from build123d import *

# Parameters (mm, degrees)
SKETCH1_W               = 298.45
SKETCH1_H               = 76.2
BOSS_EXTRUDE1_DEPTH     = 6.35
SKETCH2_W               = 12.7
SKETCH2_H               = 25.4
CUT_EXTRUDE5_DEPTH      = 155.142898393
LPATTERN1_COUNT         = 9
LPATTERN1_PITCH         = 25.4
MIRROR1_COPY_1_SKETCH_W = 12.7
MIRROR1_COPY_1_SKETCH_H = 25.4
MIRROR1_COPY_1_DEPTH    = 155.142898393
MIRROR1_COPY_2_SKETCH_W = 12.7
MIRROR1_COPY_2_SKETCH_H = 25.4
MIRROR1_COPY_2_DEPTH    = 155.142898393
MIRROR1_COPY_3_SKETCH_W = 12.7
MIRROR1_COPY_3_SKETCH_H = 25.4
MIRROR1_COPY_3_DEPTH    = 155.142898393
MIRROR1_COPY_4_SKETCH_W = 12.7
MIRROR1_COPY_4_SKETCH_H = 25.4
MIRROR1_COPY_4_DEPTH    = 155.142898393
MIRROR1_COPY_5_SKETCH_W = 12.7
MIRROR1_COPY_5_SKETCH_H = 25.4
MIRROR1_COPY_5_DEPTH    = 155.142898393
MIRROR1_COPY_6_SKETCH_W = 12.7
MIRROR1_COPY_6_SKETCH_H = 25.4
MIRROR1_COPY_6_DEPTH    = 155.142898393
MIRROR1_COPY_7_SKETCH_W = 12.7
MIRROR1_COPY_7_SKETCH_H = 25.4
MIRROR1_COPY_7_DEPTH    = 155.142898393
MIRROR1_COPY_8_SKETCH_W = 12.7
MIRROR1_COPY_8_SKETCH_H = 25.4
MIRROR1_COPY_8_DEPTH    = 155.142898393
SKETCH3_W               = 40.748476415
SKETCH3_H               = 6.35
SKETCH3_W_2             = 25.4
SKETCH3_H_2             = 9.525
CUT_EXTRUDE7_DEPTH      = 155.142898393
SKETCH4_W               = 15.875
SKETCH4_H               = 25.4
CUT_EXTRUDE8_DEPTH      = 155.142898393


with BuildPart() as part:
    # Sketch1 → Boss-Extrude1 (new body)
    with BuildSketch(Plane.XY):
        Rectangle(SKETCH1_W, SKETCH1_H)
    extrude(amount=BOSS_EXTRUDE1_DEPTH)

    # Sketch2 → Cut-Extrude5 (cut, symmetric)
    with BuildSketch(Plane.XY):
        with Locations((101.6, -44.45)):
            Rectangle(SKETCH2_W, SKETCH2_H)
    cut_extrude5 = extrude(amount=CUT_EXTRUDE5_DEPTH, both=True, mode=Mode.SUBTRACT)

    # LPattern1: Cut-Extrude5 ×9
    with Locations(*[(-i * LPATTERN1_PITCH, 0, 0) for i in range(1, LPATTERN1_COUNT)]):
        add(cut_extrude5, mode=Mode.SUBTRACT)

    # Mirror1: Cut-Extrude5 across plane
    add(cut_extrude5.mirror(Plane.ZX), mode=Mode.SUBTRACT)

    # Mirror1 copy 1 sketch → Mirror1 copy 1 (cut, symmetric)
    with BuildSketch(Plane(origin=(-25.4, 0, 0), x_dir=(1, 0, 0), z_dir=(0, 0, 1))):
        with Locations((101.6, 44.45)):
            Rectangle(MIRROR1_COPY_1_SKETCH_W, MIRROR1_COPY_1_SKETCH_H)
    extrude(amount=MIRROR1_COPY_1_DEPTH, both=True, mode=Mode.SUBTRACT)

    # Mirror1 copy 2 sketch → Mirror1 copy 2 (cut, symmetric)
    with BuildSketch(Plane(origin=(-50.8, 0, 0), x_dir=(1, 0, 0), z_dir=(0, 0, 1))):
        with Locations((101.6, 44.45)):
            Rectangle(MIRROR1_COPY_2_SKETCH_W, MIRROR1_COPY_2_SKETCH_H)
    extrude(amount=MIRROR1_COPY_2_DEPTH, both=True, mode=Mode.SUBTRACT)

    # Mirror1 copy 3 sketch → Mirror1 copy 3 (cut, symmetric)
    with BuildSketch(Plane(origin=(-76.2, 0, 0), x_dir=(1, 0, 0), z_dir=(0, 0, 1))):
        with Locations((101.6, 44.45)):
            Rectangle(MIRROR1_COPY_3_SKETCH_W, MIRROR1_COPY_3_SKETCH_H)
    extrude(amount=MIRROR1_COPY_3_DEPTH, both=True, mode=Mode.SUBTRACT)

    # Mirror1 copy 4 sketch → Mirror1 copy 4 (cut, symmetric)
    with BuildSketch(Plane(origin=(-101.6, 0, 0), x_dir=(1, 0, 0), z_dir=(0, 0, 1))):
        with Locations((101.6, 44.45)):
            Rectangle(MIRROR1_COPY_4_SKETCH_W, MIRROR1_COPY_4_SKETCH_H)
    extrude(amount=MIRROR1_COPY_4_DEPTH, both=True, mode=Mode.SUBTRACT)

    # Mirror1 copy 5 sketch → Mirror1 copy 5 (cut, symmetric)
    with BuildSketch(Plane(origin=(-127, 0, 0), x_dir=(1, 0, 0), z_dir=(0, 0, 1))):
        with Locations((101.6, 44.45)):
            Rectangle(MIRROR1_COPY_5_SKETCH_W, MIRROR1_COPY_5_SKETCH_H)
    extrude(amount=MIRROR1_COPY_5_DEPTH, both=True, mode=Mode.SUBTRACT)

    # Mirror1 copy 6 sketch → Mirror1 copy 6 (cut, symmetric)
    with BuildSketch(Plane(origin=(-152.4, 0, 0), x_dir=(1, 0, 0), z_dir=(0, 0, 1))):
        with Locations((101.6, 44.45)):
            Rectangle(MIRROR1_COPY_6_SKETCH_W, MIRROR1_COPY_6_SKETCH_H)
    extrude(amount=MIRROR1_COPY_6_DEPTH, both=True, mode=Mode.SUBTRACT)

    # Mirror1 copy 7 sketch → Mirror1 copy 7 (cut, symmetric)
    with BuildSketch(Plane(origin=(-177.8, 0, 0), x_dir=(1, 0, 0), z_dir=(0, 0, 1))):
        with Locations((101.6, 44.45)):
            Rectangle(MIRROR1_COPY_7_SKETCH_W, MIRROR1_COPY_7_SKETCH_H)
    extrude(amount=MIRROR1_COPY_7_DEPTH, both=True, mode=Mode.SUBTRACT)

    # Mirror1 copy 8 sketch → Mirror1 copy 8 (cut, symmetric)
    with BuildSketch(Plane(origin=(-203.2, 0, 0), x_dir=(1, 0, 0), z_dir=(0, 0, 1))):
        with Locations((101.6, 44.45)):
            Rectangle(MIRROR1_COPY_8_SKETCH_W, MIRROR1_COPY_8_SKETCH_H)
    extrude(amount=MIRROR1_COPY_8_DEPTH, both=True, mode=Mode.SUBTRACT)

    # Sketch3 → Cut-Extrude7 (cut, through all)
    with BuildSketch(Plane.XY):
        with Locations((163.249238208, 12.7)):
            Rectangle(SKETCH3_W, SKETCH3_H)
        with Locations((163.249238208, 0)):
            Rectangle(SKETCH3_W, SKETCH3_H)
        with Locations((163.249238208, -12.7)):
            Rectangle(SKETCH3_W, SKETCH3_H)
        with Locations((155.575, 26.9875)):
            Rectangle(SKETCH3_W_2, SKETCH3_H_2)
        with Locations((155.575, -26.9875)):
            Rectangle(SKETCH3_W_2, SKETCH3_H_2)
    cut_extrude7 = extrude(amount=CUT_EXTRUDE7_DEPTH, mode=Mode.SUBTRACT)

    # Mirror2: Cut-Extrude7 across plane
    add(cut_extrude7.mirror(Plane(origin=(0, 0, 0), x_dir=(0, 0, 1), z_dir=(1, 0, 0))), mode=Mode.SUBTRACT)

    # Sketch4 → Cut-Extrude8 (cut, through all)
    with BuildSketch(Plane.XY.offset(6.35)):
        with Locations((128.5875, -44.45)):
            Rectangle(SKETCH4_W, SKETCH4_H)
        with Locations((-128.5875, -44.45)):
            Rectangle(SKETCH4_W, SKETCH4_H)
        with Locations((-128.5875, 44.45)):
            Rectangle(SKETCH4_W, SKETCH4_H)
        with Locations((128.5875, 44.45)):
            Rectangle(SKETCH4_W, SKETCH4_H)
    extrude(amount=-CUT_EXTRUDE8_DEPTH, mode=Mode.SUBTRACT)


solid = part.part
Work out the finished part from the listing and answer in its coordinate system (mm). A direction names the side the tool comes from. Give positions to 0.01 mm unless a question says otherwise; leave off trailing zeros. Loops run counter-clockwise (first coordinate to the right, second up) from the corner with the lowest first, then second, coordinate; pieces in that order, holes last. Notation, with made-up numbers: (-3, -25.5) -> (19, -25.5) arc R17 cw to (19, 2.5) -> close; hole circle Ø1 at (-25.75, 4). An arc over 180 degrees is marked (long way). Use a Markdown table: item, result. Add a question column.
1. Section A-A on y = -12.5 is taken. Determine the outline of the cut face in (x, z) (3 decimals).
2. Section B-B on x = 28.5 is taken. Determine the outline of the cut face in (y, z), and give its area (3 significant figures).
3. For faces 1 (the flat face through (146, -3.175, 3)), 2 (the flat face through (95.25, 35, 3)), 3 (the flat face through (-25, -31.75, 3)), 4 (the flat face through (-146, 22.225, 3)), determine the directions among +Z, -Z, +X, -X, +Y, -Y from which every point of the face is accessible in a straight line to the end or side of a thin tool.
4. Find the intervals of material crossed by probe 1 along Y at (x, z) = (-3.5, 3.75); probe 2 along X at (y, z) = (30.5, 5) (3 decimals), in increasing order.
5. Flat-ended cylindrical pins translate along their axes: pin 1 Ø3 at (x, y) = (24.5, -14) entering from -Z; pin 2 Ø3 at (x, z) = (-126.5, 4) entering from +Y; pin 3 Ø3 at (x, z) = (-124.5, 2) entering from -Y. Find the tip coordinate at first contact, or state that the pin passes through.
6. Determine the mould class of faces 5 (the flat face through (149.225, 19, 3)), 6 (the flat face through (-25, 31.75, 3)), 7 (the flat face through (-19.05, -35, 3)), 8 (the flat face through (-146, 9.525, 3)) for opening direction X: released by +X, released by -X, zero draft, split by the parting line, or undercut.
Results below:
| question | item | result |
|---|---|---|
| 1 | outline | (-142.875, 0) -> (142.875, 0) -> (142.875, 6.35) -> (-142.875, 6.35) -> close |
| 2 | outline | (-31.75, 0) -> (31.75, 0) -> (31.75, 6.35) -> (-31.75, 6.35) -> close |
| 2 | area | 403 mm^2 |
| 3 | face 1 | +Z, -Z, +X |
| 3 | face 2 | +Z, -Z, +Y |
| 3 | face 3 | +Z, -Z, -Y |
| 3 | face 4 | +Z, -Z, -X |
| 4 | probe 1 | y = -31.75 to 31.75 |
| 4 | probe 2 | x = -142.875 to 142.875 |
| 5 | pin 1 | stops at z = 0 |
| 5 | pin 2 | stops at y = 31.75 |
| 5 | pin 3 | stops at y = -31.75 |
| 6 | face 5 | released by +X |
| 6 | face 6 | undercut |
| 6 | face 7 | undercut |
| 6 | face 8 | zero draft |
